Geometry check sheet. Reference: the model listing, model coordinates, mm. Face numbers are marked on the shaded views. A direction names the side the tool comes from. Give positions to 0.01 mm unless a question says otherwise; leave off trailing zeros. Order: outer loops, then holes, each group sorted by start corner. A loop starts at its lowest first (then second) coordinate and runs counter-clockwise, first axis right, second up.
from build123d import *

# Parameters (mm, degrees)
BOSS_EXTRUDE1_DEPTH   = 4
BOSS_EXTRUDE1_2_DEPTH = 4
SKETCH3_W             = 10
SKETCH3_H             = 6.473357475
SKETCH3_W_2           = 50.25
BOSS_EXTRUDE3_DEPTH   = 4
FILLET2_R             = 1
SKETCH4_W             = 14.347682942
SKETCH4_H             = 10
BOSS_EXTRUDE4_DEPTH   = 15
SKETCH6_W             = 14.347682942
SKETCH6_H             = 3
BOSS_EXTRUDE6_DEPTH   = 10
CUT_EXTRUDE1_REACH    = 55.674
SKETCH7_R             = 1.325
SKETCH8_W             = 16.45797352
SKETCH8_H             = 4
SKETCH8_H_2           = 11.134864375
SKETCH8_R             = 1.8
BOSS_EXTRUDE7_DEPTH   = 5


with BuildPart() as part:
    # Sketch1 → Boss-Extrude1 (new body)
    with BuildSketch(Plane(origin=(0, 0, 0), x_dir=(1, 0, 0), z_dir=(0, 1, 0))):
        with BuildLine():
            Line((-23.6, 10.542278437), (-17, 10.542278437))
            ThreePointArc((-17, 10.542278437), (-15.475, 9.017278437), (-17, 7.492278437))
            Line((-17, 7.492278437), (-23.6, 7.492278437))
            ThreePointArc((-23.6, 7.492278437), (-25.125, 9.017278437), (-23.6, 10.542278437))
        make_face()
    extrude(amount=BOSS_EXTRUDE1_DEPTH)



with BuildPart() as body_2:
    # Sketch1 → Boss-Extrude1 2 (new body)
    with BuildSketch(Plane(origin=(0, 0, 0), x_dir=(1, 0, 0), z_dir=(0, 1, 0))):
        with BuildLine():
            Line((23.6, 7.492278437), (17, 7.492278437))
            ThreePointArc((17, 7.492278437), (15.475, 9.017278437), (17, 10.542278437))
            Line((17, 10.542278437), (23.6, 10.542278437))
            ThreePointArc((23.6, 10.542278437), (25.125, 9.017278437), (23.6, 7.492278437))
        make_face()
    extrude(amount=BOSS_EXTRUDE1_2_DEPTH)


with BuildPart() as part_1:
    add(part.part)

    add(body_2.part)  # Boss-Extrude3 merges body 2
    # Sketch3 → Boss-Extrude3 (add)
    with BuildSketch(Plane(origin=(0, 4, 0), x_dir=(1, 0, 0), z_dir=(0, 1, 0))):
        with Locations((-30.125, 30.8805997)):
            Rectangle(SKETCH3_W, SKETCH3_H)
        with Locations((0, 30.8805997)):
            Rectangle(SKETCH3_W_2, SKETCH3_H)
        with BuildLine():
            Line((25.125, 27.643920962), (-25.125, 27.643920962))
            Line((-25.125, 27.643920962), (-25.125, 18.723444743))
            Line((-25.125, 18.723444743), (-25.125, 9.017278437))
            ThreePointArc((-25.125, 9.017278437), (-24.678337841, 7.938940596), (-23.6, 7.492278437))
            Line((-23.6, 7.492278437), (-17, 7.492278437))
            ThreePointArc((-17, 7.492278437), (-15.921662159, 7.938940596), (-15.475, 9.017278437))
            Line((-15.475, 9.017278437), (-15.475, 14.117278437))
            Line((-15.475, 14.117278437), (15.475, 14.117278437))
            Line((15.475, 14.117278437), (15.475, 9.017278437))
            ThreePointArc((15.475, 9.017278437), (15.921662159, 7.938940596), (17, 7.492278437))
            Line((17, 7.492278437), (23.6, 7.492278437))
            ThreePointArc((23.6, 7.492278437), (24.678337841, 7.938940596), (25.125, 9.017278437))
            Line((25.125, 9.017278437), (25.125, 18.723444743))
            Line((25.125, 18.723444743), (25.125, 27.643920962))
        make_face()
    extrude(amount=BOSS_EXTRUDE3_DEPTH)

    # Fillet2
    fillet2_edges = [part_1.edges().sort_by_distance(p)[0] for p in [
        (-25.125, 8, -18.3305997),
        (15.475, 8, -11.567278437),
        (-24.678337841, 8, -7.938940596),
        (-20.3, 8, -7.492278437),
        (-15.921662159, 8, -7.938940596),
        (-15.475, 8, -11.567278437),
        (15.921662159, 8, -7.938940596),
        (20.3, 8, -7.492278437),
        (24.678337841, 8, -7.938940596),
        (25.125, 8, -21.567278437),
    ]]
    fillet(fillet2_edges, radius=FILLET2_R)

    # Sketch4 → Boss-Extrude4 (add)
    with BuildSketch(Plane(origin=(0, 8, 0), x_dir=(1, 0, 0), z_dir=(0, 1, 0))):
        with Locations((-7.885296824, 29.117278437)):
            Rectangle(SKETCH4_W, SKETCH4_H)
    extrude(amount=BOSS_EXTRUDE4_DEPTH)

    # Sketch6 → Boss-Extrude6 (add)
    with BuildSketch(Plane(origin=(0, 23, 0), x_dir=(1, 0, 0), z_dir=(0, 1, 0))):
        with Locations((-7.885296824, 32.617278437)):
            Rectangle(SKETCH6_W, SKETCH6_H)
    extrude(amount=BOSS_EXTRUDE6_DEPTH)

    # Sketch7 → Cut-Extrude1 (cut, up to next)
    with BuildSketch(Plane.XY.offset(-31.117278437), mode=Mode.PRIVATE) as cut_extrude1_sk1:
        with Locations((-11.819138295, 29.375)):
            Circle(SKETCH7_R)
    cut_extrude1_tool1 = extrude(cut_extrude1_sk1.sketch, amount=-CUT_EXTRUDE1_REACH, mode=Mode.PRIVATE) & part_1.part
    # Sketch7 → Cut-Extrude1 (cut, up to next)
    with BuildSketch(Plane.XY.offset(-31.117278437), mode=Mode.PRIVATE) as cut_extrude1_sk2:
        with Locations((-5.789138295, 29.375)):
            Circle(SKETCH7_R)
    cut_extrude1_tool2 = extrude(cut_extrude1_sk2.sketch, amount=-CUT_EXTRUDE1_REACH, mode=Mode.PRIVATE) & part_1.part
    add(cut_extrude1_tool1.solids().sort_by_distance((-11.819138, 29.375, -31.117278))[0], mode=Mode.SUBTRACT)
    add(cut_extrude1_tool2.solids().sort_by_distance((-5.789138, 29.375, -31.117278))[0], mode=Mode.SUBTRACT)

    # Sketch8 → Boss-Extrude7 (add)
    # profile 1 of 2: a face of its own
    with BuildSketch(Plane(origin=(0, 0, -34.117278437), x_dir=(-1, 0, 0), z_dir=(0, 0, -1))):
        with Locations((26.89601324, 6)):
            Rectangle(SKETCH8_W, SKETCH8_H)
    # profile 2 of 2: a face of its own
    with BuildSketch(Plane(origin=(0, 0, -34.117278437), x_dir=(-1, 0, 0), z_dir=(0, 0, -1))):
        with Locations((26.89601324, -1.567432188)):
            Rectangle(SKETCH8_W, SKETCH8_H_2)
        with Locations((22.984760942, -0.83124894)):
            Circle(SKETCH8_R, mode=Mode.SUBTRACT)
        with Locations((30.984760942, -0.83124894)):
            Circle(SKETCH8_R, mode=Mode.SUBTRACT)
    extrude(amount=-BOSS_EXTRUDE7_DEPTH)


solid = part_1.part
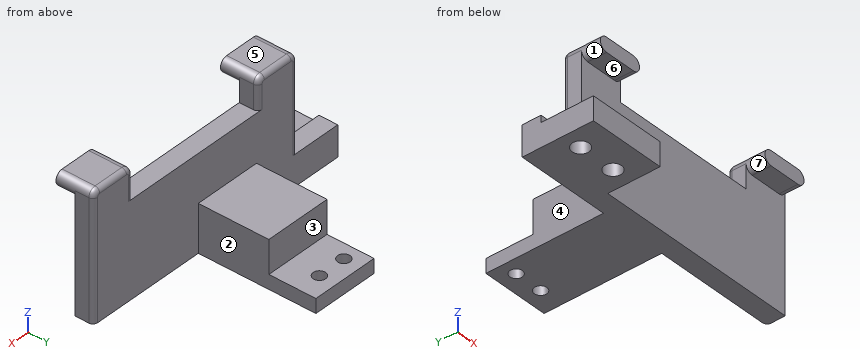
Item 1: Gauge pin test, flat ends, axial feed: pin 1 (5.5 mm diameter, centred on x = -9.5, z = -27, fed in from +Y); pin 2 (1.5 mm diameter, centred on y = 5, z = -22.5, fed in from -X) (3 decimals); pin 3 (3 mm diameter, centred on y = 16, z = -23.5, fed in from +X); pin 4 (3 mm diameter, centred on x = -30.98, y = -0.83, fed in from -Z). Record the tip position at first contact, or that the pin passes through.
Reported:
pin 1: stops at y = 23
pin 2: stops at x = -25.125
pin 3: stops at x = -0.71
pin 4: passes through
Item 2: Scan lines: L1, parallel to Y at x = 18.5, z = -10; L2, parallel to Y at x = -6.5, z = -19.5; L3, parallel to X at y = 5, z = -20 (3 decimals). Record each from-to range of solid material in increasing order.
Reported:
L1: y = 0 to 8
L2: y = 4 to 8
L3: x = -25.125 to 25.125
Item 3: Set-up check for the marked faces 1, 2 and 3: record each of +Z, -Z, +X, -X, +Y, -Y from which the full face is reachable in a straight line by a thin tool's end or side.
Reported:
face 1: -X, -Y
face 2: +Z, -Z, +X, +Y
face 3: +Z, +X, -X, +Y
Item 4: Sectioned sample at C-C (z = -18.5). Enter the section's corners in (x, y) (3 decimals), and give its area (3 significant figures).
Reported:
outline: (-25.125, 4) - (25.125, 4) - (25.125, 7) arc R1 ccw to (24.125, 8) - (-24.125, 8) arc R1 ccw to (-25.125, 7) - close
area: 201 mm2
Item 5: Sectioned sample at B-B (x = 19). Enter the section's corners in (y, z), and give its area (3 significant figures).
Reported:
outline: (0, -10.54) - (4, -10.54) - (4, -34.12) - (8, -34.12) - (8, -8.49) arc R1 ccw to (7, -7.49) - (0, -7.49) - close
area: 118 mm2
Item 6: Sectioned sample at A-A (z = -11.5). Enter the section's corners in (x, y) (3 decimals).
Reported:
outline: (-25.125, 4) - (-15.475, 4) - (-15.475, 7) arc R1 ccw to (-16.475, 8) - (-24.125, 8) arc R1 ccw to (-25.125, 7) - close; (15.475, 4) - (25.125, 4) - (25.125, 7) arc R1 ccw to (24.125, 8) - (16.475, 8) arc R1 ccw to (15.475, 7) - close
Item 7: Draft check along Z on the marked faces 4, 5, 6 and 7. Enter one of: released by +Z, released by -Z, zero draft, split by the parting line, or undercut.
Reported:
face 4: zero draft
face 5: released by +Z
face 6: undercut
face 7: split by the parting line
Item 8: Sectioned sample at D-D (y = 27). Enter the section's corners in (x, z).
Reported:
outline: (-15.06, -34.12) - (-0.71, -34.12) - (-0.71, -31.12) - (-15.06, -31.12) - close
